The listing builds one solid part. Answer for the finished solid, in the listing's coordinates (mm). A direction names the side the tool comes from. Round coordinates to 2 decimals unless told otherwise and drop trailing zeros. Write each loop counter-clockwise with the first axis right and the second up, starting at its lowest first coordinate (ties: lowest second). Pieces come first, ordered by that corner, then holes.
Item 1: Find section A-A on z = 17.5. Give the vertices of the cut face in (x, y), then the cut area to 3 significant figures.
Item 2: Each of these flat-tipped pins is pushed along its axis until it touches: pin 1 (12 mm diameter, centred on y = 52, z = 60, fed in from -X); pin 2 (5 mm diameter, centred on x = 3, y = 37.5, fed in from -Z); pin 3 (1.5 mm diameter, centred on x = 25, z = 2.5, fed in from +Y); pin 4 (5 mm diameter, centred on x = 3, y = 55, fed in from +Z). Where does it stop, or does it pass through?
Item 3: Find section D-D on x = 1.5. Give the vertices of the cut face in (y, z), then the cut area to 3 significant figures.
Item 4: Find section B-B on x = 47. Give the vertices of the cut face in (y, z).
Item 5: Find the intervals of material crossed by probe 1 along Y at (x, z) = (0, 3); probe 2 along Y at (x, z) = (45, 16); probe 3 along Z at (x, y) = (-7.5, 7.5), in increasing order.
Item 6: For a pull along Y with two mould halves and no side action, classify faces 4 (the face through (-1.658, -7.468, 2.465)), 5 (the face through (-15, 24, 2)), 6 (the face through (43, 35, 15)) as +Y half, -Y half, draft (parallel to the pull), parting line (faces both ways), or undercut.
Item 7: Find section C-C on y = 40.5. Give the vertices of the cut face in (x, z), then the cut area to 4 significant figures.
Item 8: A tool of negligible diameter and unlimited length cuts with its end or side. For faces 1 (the face through (30, 43, 15)), 2 (the face through (58, 26, 105)), 3 (the face through (22, 50, 2)), from which of +Z, -Z, +X, -X, +Y, -Y can it reach the whole face along a straight path? Write none if from no direction.
```python
from build123d import *

# Parameters (mm, degrees)
SKETCH1_R           = 7.65
BOSS_EXTRUDE2_DEPTH = 5
SKETCH2_W           = 3
SKETCH2_H           = 80
BOSS_EXTRUDE3_DEPTH = 100
SKETCH3_R           = 7.65
BOSS_EXTRUDE4_DEPTH = 20


with BuildPart() as part:
    # Sketch1 → Boss-Extrude2 (new body)
    with BuildSketch(Plane.XY):
        with BuildLine():
            Line((-15, 65), (0, 65))
            ThreePointArc((0, 65), (10.606601718, 60.606601718), (15, 50))
            Line((15, 50), (30, 50))
            ThreePointArc((30, 50), (34.393398282, 60.606601718), (45, 65))
            Line((45, 65), (60, 65))
            Line((60, 65), (60, 41.966335985))
            Line((60, 41.966335985), (60, -15))
            Line((60, -15), (12.652076701, -15))
            Line((12.652076701, -15), (-15, -15))
            Line((-15, -15), (-15, 65))
        make_face()
        Circle(SKETCH1_R, mode=Mode.SUBTRACT)
        with Locations((45, 50)):
            Circle(SKETCH1_R, mode=Mode.SUBTRACT)
        with Locations((0, 50)):
            Circle(SKETCH1_R, mode=Mode.SUBTRACT)
    extrude(amount=BOSS_EXTRUDE2_DEPTH)

    # Sketch2 → Boss-Extrude3 (add)
    with BuildSketch(Plane.XY.offset(5)):
        with Locations((58.5, 25)):
            Rectangle(SKETCH2_W, SKETCH2_H)
    extrude(amount=BOSS_EXTRUDE3_DEPTH)

    # Sketch3 → Boss-Extrude4 (add)
    with BuildSketch(Plane.XY.offset(5)):
        with BuildLine():
            Line((30, 50), (30, 35))
            Line((30, 35), (57, 35))
            Line((57, 35), (57, 65))
            Line((57, 65), (45, 65))
            ThreePointArc((45, 65), (34.393398282, 60.606601718), (30, 50))
        make_face()
        with Locations((45, 50)):
            Circle(SKETCH3_R, mode=Mode.SUBTRACT)
    extrude(amount=BOSS_EXTRUDE4_DEPTH)


solid = part.part
```
Check values:
1. outline: (30, 35) - (57, 35) - (57, -15) - (60, -15) - (60, 65) - (45, 65) arc R15 ccw to (30, 50) - close; hole circle Ø15.3 at (45, 50)
1. area: 818 mm2
2. pin 1: stops at x = 57
2. pin 2: stops at z = 0
2. pin 3: stops at y = 50
2. pin 4: stops at z = 5
3. outline: (-15, 0) - (-7.5, 0) - (-7.5, 5) - (-15, 5) - close; (7.5, 0) - (42.5, 0) - (42.5, 5) - (7.5, 5) - close; (57.5, 0) - (64.92, 0) - (64.92, 5) - (57.5, 5) - close
3. area: 250 mm2
4. outline: (-15, 0) - (42.62, 0) - (42.62, 25) - (35, 25) - (35, 5) - (-15, 5) - close; (57.38, 0) - (65, 0) - (65, 25) - (57.38, 25) - close
5. probe 1: y = -15 to -7.65, 7.65 to 42.35, 57.65 to 65
5. probe 2: y = 35 to 42.35, 57.65 to 65
5. probe 3: z = 0 to 5
6. face 4: undercut
6. face 5: draft
6. face 6: -Y half
7. outline: (-15, 0) - (60, 0) - (60, 105) - (57, 105) - (57, 25) - (30, 25) - (30, 5) - (-15, 5) - close
7. area: 1,215 mm2
8. face 1: +Z, -X, +Y, -Y
8. face 2: +Z, +X, -X, +Y, -Y
8. face 3: +Z, -Z, +Y
